For this review, take the finished solid that the model builds, in its own axes (mm). A direction names the side the tool comes from. Coordinates: 2 decimals unless noted, no trailing zeros. Loops run counter-clockwise (first coordinate to the right, second up) from the corner with the lowest first, then second, coordinate; pieces in that order, holes last. Notation, with made-up numbers: M -35.75,87 L -31.75,87 A24 ccw -31.75,109 Z; hole C -31,37 d6. An arc over 180 degrees is marked long. Use one line per item in the form item = value.
Autodesk Inventor part; units mm, degrees
ref_plane "YZ Plane" through (0, 0, 0) normal (1, 0, 0) x (0, 1, 0)
ref_plane "XZ Plane" through (0, 0, 0) normal (0, 1, 0) x (-1, 0, 0)
ref_plane "XY Plane" through (0, 0, 0) normal (0, 0, 1) x (1, 0, 0)
sketch "Sketch2" plane through (0, 0, 0) normal (1, 0, 0) x (0, 1, 0)
  line L0 (0, 0) -> (19.05, 0)
  line L1 (19.05, 0) -> (19.05, -6.35)
  line L2 (19.05, -6.35) -> (0, -6.35)
  line L3 (0, -6.35) -> (0, 0)
  line L4 (0, 0) -> (19.05, 0)
  line L5 (19.05, 0) -> (19.05, -20.6375)
  line L6 (19.05, -20.6375) -> (0, -20.6375)
  line L7 (0, -20.6375) -> (0, 0)
  line L8 (0, -16.7624) -> (10.3188, -16.7624) construction
  line L9 (10.3188, -16.7624) -> (10.3188, -6.35)
  line L10 (10.3188, -6.35) -> (0, -6.35)
  line L11 (0, -6.35) -> (0, -16.7624)
  line L12 (10.3188, -16.7624) -> (0, -19.05)
  line L13 (6.35, -20.6375) -> (19.05, -17.4625)
  line L14 (19.05, 0) -> (12.05, 0)
  line L15 (12.05, 0) -> (12.05, -13.975)
  line L16 (12.05, -13.975) -> (19.05, -13.975)
  line L17 (19.05, -13.975) -> (19.05, 0)
  line L18 (10.3188, -15.0812) -> (4.7625, -15.0812)
  line L19 (4.7625, -15.0812) -> (4.7625, -6.35)
  line L20 (4.7625, -6.35) -> (10.3188, -6.35)
  line L21 (10.3188, -6.35) -> (10.3188, -15.0812)
  line L22 (4.7625, -9.525) -> (10.3188, -15.0812)
  line L23 (19.05, 0) -> (23.8125, 0)
  line L24 (23.8125, 0) -> (23.8125, -20.6375)
  line L25 (23.8125, -20.6375) -> (19.05, -20.6375)
  line L26 (19.05, -20.6375) -> (19.05, 0)
  line L27 (23.8125, 0) -> (19.8125, 0)
  line L28 (19.8125, 0) -> (19.8125, -18.5)
  line L29 (19.8125, -18.5) -> (23.8125, -18.5)
  line L30 (23.8125, -18.5) -> (23.8125, 0)
  line L31 (19.8125, -17.4625) -> (19.05, -17.4625)
  line L32 (12.05, -12.7) -> (10.3188, -6.35)
  line L33 (10.3188, -6.35) -> (8.3344, -6.35)
  line L34 (8.3344, -6.35) -> (8.3344, -5.5562)
  line L35 (8.3344, -5.5562) -> (10.3188, -5.5562)
  line L36 (10.3188, -5.5562) -> (10.3188, -6.35)
  point P0 (19.05, -13.975)
  point P1 (12.05, -6.35)
  point P2 (4.7625, -6.35)
  point P3 (12.05, 0)
  point P4 (23.8125, -18.5)
  point P5 (10.3188, -6.35)
  point P6 (10.3188, -6.35)
  dimension "d4" = 19.05
  dimension "d5" = 6.35
  dimension "d6" = 20.6375
  dimension "d7" = 12.5
  dimension "d9" = 10.3187
  dimension "d11" = 19.05
  dimension "d35" = 6.35
  dimension "d36" = 7
  dimension "d37" = 13.975
  dimension "d38" = 17.4625
  dimension "d41" = 4.7625
  dimension "d42" = 5.5563
  dimension "d43" = 3.175
  dimension "d54" = 4.7625
  dimension "d55" = 4
  dimension "d56" = 18.5
  dimension "d57" = 12.7
  dimension "d58" = 1.9844
  dimension "d59" = 0.7937
revolve "Revolution1" add sketch "Sketch2" angle 360 about axis through (0, 0, 0) along (0, 1, 0) contours L2 L9 L22 L19 | L32 L15 L16 L5 L13 L6 L7 L12 L9 | L2 L34 L35 L36 | L28 L29 L24 L25 L5 L31 | L5 L6 L13
chamfer "Chamfer1" distance 0.3969 angle 45 3 edges at (0, 0, 20.6375) (0, 4.7625, 9.525) (0, 23.8125, 20.6375)
thicken "Thicken1" operation cut thickness 0.1 both sides no extend neighbours no toward (0.1604113, 0, -0.9870503) faces at (2.9676, 22.4792, -18.2604)
thicken "Thicken2" operation cut thickness 0.1 both sides no extend neighbours no toward (0.0804666, 0, -0.9967573) faces at (1.1245, 16.7167, -13.9297)
thicken "Thicken4" operation add thickness 0.1 both sides no extend neighbours yes toward (0.0804666, 0, -0.9967573) faces at (0.511, 5.9531, -6.3294)
properties part number "Flywheel" material "Brass, Soft Yellow"
1. Wall thickness on line 1 along Z through (x, y) = (0.5, 21.5); line 2 along X through (y, z) = (19.55, 0); line 3 along X through (y, z) = (7.55, 0): over which ranges is each line inside the solid? List them lowest first. Write a range as from..to.
Computed values:
line_1 = -20.63..-18.59, 18.59..20.63
line_2 = -20.64..-17.46, 17.46..20.64
line_3 = -20.64..-17.38, -12.31..-6.45, 6.45..12.31, 17.38..20.64
2. Consider section C-C on y = 9.5. Write out the cut boundary in (x, z) (1 decimal), plus the area to 3 significant figures.
Computed values:
outline = C 0,0 d41.3; C 0,0 d28.5; hole C 0,0 d33.9; hole C 0,0 d11.1
area = 978 mm2
3. Consider section A-A on y = 6. State how many separate pieces and enclosed holes the cut face has, plus the area to 3 significant figures.
Computed values:
separate_pieces = 2
enclosed_holes = 2
area = 585 mm2
4. For pin 1 Ø17 at (x, z) = (0, 0) entering from -Y; pin 2 Ø20.5 at (x, z) = (0, 0) entering from +Y; pin 3 Ø6.5 at (x, z) = (-2, 1) entering from +Y; pin 4 Ø8 at (y, z) = (17.5, 0.5) entering from -X, all flat-tipped, find the tip position at first contact; note any pin that passes through.
Computed values:
pin_1 = 4.76
pin_2 = 11.38
pin_3 = through
pin_4 = -20.64
5. Tool access review of faces 4 (the face through (13.74, 15.6, 3.05)), 5 (the face through (-6, 10.319, 14)), 6 (the face through (3.38, 9.34, 4.41)): name each direction out of +Z, -Z, +X, -X, +Y, -Y from which nothing blocks a thin tool from reaching the whole face with its end or side.
Computed values:
face_4 = +Y
face_5 = -Y
face_6 = +Y, -Y
6. Draft analysis for pull direction Z (two halves, no side actions). For faces 1 (the face through (6, 4.762, -4)), 2 (the face through (-20.147, 11.745, 4.474)), 3 (the face through (12, 0, -15)), state which applies: +Z half, -Z half, draft (parallel to the pull), parting line (faces both ways), or undercut.
Computed values:
face_1 = undercut
face_2 = parting line
face_3 = draft
